Could you check a few things on this model? Use its own coordinates, in mm. A direction names the side the tool comes from. Give positions to 0.01 mm unless a question says otherwise; leave off trailing zeros. Order: outer loops, then holes, each group sorted by start corner. A loop starts at its lowest first (then second) coordinate and runs counter-clockwise, first axis right, second up.
Autodesk Inventor part; units mm, degrees
ref_plane "YZ Plane" through (0, 0, 0) normal (1, 0, 0) x (0, 1, 0)
ref_plane "XZ Plane" through (0, 0, 0) normal (0, 1, 0) x (-1, 0, 0)
ref_plane "XY Plane" through (0, 0, 0) normal (0, 0, 1) x (1, 0, 0)
sketch "Skizze1" plane through (0, 0, 0) normal (0, 0, 1) x (1, 0, 0)
  circle A0 centre (0, 0) radius 34
  dimension "d0" = 68
extrude "Extrusion1" add sketch "Skizze1" along normal mid plane 21
sketch "Skizze2" plane through (0, 0, 10.5) normal (0, 0, 1) x (1, 0, 0)
  circle A0 centre (0, 0) radius 30
  dimension "d3" = 60
extrude "Extrusion2" cut sketch "Skizze2" against normal blind 3
fillet "Rundung1" radius 2 1 edges at (-30, 0, 7.5)
sketch "Skizze3" plane through (0, 0, -10.5) normal (0, 0, -1) x (-1, 0, 0)
  circle A0 centre (0, 0) radius 30
  dimension "d7" = 60
extrude "Extrusion3" cut sketch "Skizze3" against normal blind 10
fillet "Rundung2" radius 2 1 edges at (30, 0, -0.5)
sketch "Skizze4" plane through (0, 0, -0.5) normal (0, 0, -1) x (-1, 0, 0)
  circle A0 centre (0, 0) radius 8
  dimension "d11" = 16
extrude "Extrusion4" add sketch "Skizze4" along normal blind 3.5
sketch "Skizze5" plane through (0, 0, -4) normal (0, 0, -1) x (-1, 0, 0)
  circle A0 centre (0, 0) radius 8
hole "Bohrung1" at (0, 0, -4) direction (0, 0, 1) diameter 10 depth 11.5
sketch "Skizze6" plane through (0, 0, -0.5) normal (0, 0, -1) x (-1, 0, 0)
  circle A0 centre (0, 0) radius 8
  line L0 (0, 0) -> (0, 46.0089) construction
  circle A1 centre (0, 0) radius 5
  line L1 (0, 0) -> (-23.7907, 41.2067) construction
  circle A2 centre (0, 0) radius 19 construction
  point P0 (-9.5, 16.4545)
  dimension "d22" = 38
  dimension "d21" = 30
hole "Bohrung2" at (9.5, 16.4545, -0.5) direction (0, 0, 1) diameter 15 depth 8
pattern_circular "Runde Anordnung1" count 6 over 360 about axis through (0, 0, -10.5) along (0, 0, 1) of "Bohrung2"
sketch "Skizze7" plane through (0, 0, -10.5) normal (0, 0, -1) x (-1, 0, 0)
  point P0 (0, 0)
  point P1 (0, -31.75)
  dimension "d40" = 31.75
hole "Bohrung3" at (0, -31.75, -10.5) direction (0, 0, 1) diameter 2 end through all
sketch "Skizze8" plane through (0, 0, 7.5) normal (0, 0, 1) x (1, 0, 0)
  point P0 (0, 0)
  point P1 (0, -8.75)
  dimension "d48" = 8.75
hole "Bohrung4" at (0, -8.75, 7.5) direction (0, 0, -1) diameter 2 end through all
properties part number "schwingrad" material "Polypropylen"
Item 1: Imagine slicing it at B-B on z = 2. Give the number of separate pieces and of enclosed holes in the cut face, then the cut area to 3 significant figures.
Findings:
separate pieces: 1
enclosed holes: 9
area: 2,490 mm2
Item 2: For pin 1 (19.5 mm diameter, centred on x = -9.5, y = 16.45, fed in from -Z); pin 2 (9 mm diameter, centred on x = 19, y = 0, fed in from -Z); pin 3 (12 mm diameter, centred on x = 14.5, y = -13, fed in from -Z); pin 4 (5 mm diameter, centred on y = 8, z = 4, fed in from +X), each with a flat end and sliding along its axis, tell me the tip position at first contact or that it passes through.
Findings:
pin 1: stops at z = -0.64
pin 2: passes through
pin 3: stops at z = -0.5
pin 4: stops at x = 33.55
Item 3: We'd pull the mould along X, two halves only. Please class faces 4 (the cylindrical face through (18.28, 28.67, 0.15)), 5 (the flat face through (20, -23, -10.5)), 6 (the cylindrical face through (-29.97, 1.32, 10.01)), 7 (the flat face through (0.1, -5.2, -4)): +X half, -X half, draft (parallel to the pull), parting line (faces both ways), or undercut.
Findings:
face 4: parting line
face 5: draft
face 6: undercut
face 7: undercut
Item 4: Imagine slicing it at A-A on z = -1.5. List the corners of the cut face in (x, y) for me (3 decimals), then the cut area to 3 significant figures.
Findings:
outline: circle Ø68 at (0, 0); (-0.632, -7.975) arc R1 cw to (0.632, -7.975) arc R8 ccw (long way) to start; hole circle Ø59.464 at (0, 0); hole circle Ø10 at (0, 0); hole circle Ø2 at (0, -31.75)
area: 974 mm2
Item 5: For faces 1 (the cylindrical face through (0.383, -30.826, 0.147)), 2 (the cylindrical face through (29.97, 1.32, -6.56)), 3 (the flat face through (6, 0, 7.5)), which set-ups out of +Z, -Z, +X, -X, +Y, -Y let a thin tool reach every point of the face, with its end or its side?
Findings:
face 1: +Z, -Z
face 2: -Z
face 3: +Z
Item 6: Please list where these lines run through material, in increasing order: line 1 along Y through (x, z) = (0, -6.5); line 2 along Y through (x, z) = (0, -1.25); line 3 along X through (y, z) = (10, 5.5).
Findings:
line 1: y = -34 to -32.75, -30.75 to -30, 30 to 34
line 2: y = -34 to -32.75, -30.75 to -29.56, -7.75 to -5, 5 to 8, 29.56 to 34
line 3: x = -32.5 to -13.32, -5.68 to 5.68, 13.32 to 32.5
